For this review, take the finished solid that the model builds, in its own axes (mm). Coordinates: 2 decimals unless noted, no trailing zeros. Write each loop counter-clockwise with the first axis right and the second up, starting at its lowest first coordinate (ties: lowest second). Pieces come first, ordered by that corner, then holes. Notation, with made-up numbers: (72.25, -30) - (106.25, -30) arc R33 ccw to (106.25, -2) - close; hole circle Ø11 at (-37, 2.5). An arc over 180 degrees is marked (long way). Use one line per item in the form item = value. Start each with the question number.
1) Insertion check: P1, Ø1.5, axis at x = -363, z = 7.5, coming from the -Y side; P2, Ø4, axis at y = -68.5, z = 3.5, coming from the +X side. Each pin has a flat end and moves straight along its axis. Give the tip position at first contact, or say it passes through.
2) We need section A-A (z = 9). Give the boundary of the cut face in (x, y), plus the area to 3 significant figures.
3) For L1, parallel to X at y = -31, z = 15; L2, parallel to Y at x = -260, z = 17.5; L3, parallel to X at y = -38, z = 15.5, list the stretches that pass through material, from the lowest coordinate up. Write a range as from..to.
4) We need section B-B (y = -11.5). Give the boundary of the cut face in (x, z).
```python
from build123d import *

# Parameters (mm, degrees)
F0_W     = 685.8
F0_H     = 19.05
F1_DEPTH = 88.9
F3_DEPTH = 127
F5_DEPTH = 127
F7_DEPTH = 25.4


with BuildPart() as f1:
    # F0 (on Front) → F1 (new body)
    with BuildSketch(Plane.XZ):
        with Locations((-342.9, 9.525)):
            Rectangle(F0_W, F0_H)
    extrude(amount=F1_DEPTH)

    # F2 (on face) → F3 (cut)
    with BuildSketch(Plane.XY.offset(19.05)):
        Polygon((0, -88.9), (0, 0), (-62.2484501468, -88.9), align=None)
    extrude(amount=-F3_DEPTH, mode=Mode.SUBTRACT)

    # F4 (on face) → F5 (cut)
    with BuildSketch(Plane.XY.offset(19.05)):
        Polygon((-685.8, 0), (-685.8, -88.9), (-623.5515498532, 0), align=None)
    extrude(amount=-F5_DEPTH, mode=Mode.SUBTRACT)

    # F6 (on face) → F7 (cut)
    with BuildSketch(Plane.XY.offset(19.05)):
        Polygon((-685.8, -88.9), (-62.2484501468, -88.9), (-54.6331555624, -78.0242322185), (-659.9736535614, -52.0161548124), align=None)
    extrude(amount=-F7_DEPTH, mode=Mode.SUBTRACT)


solid = f1.part
```
Determined:
q1.P1 = -64.81
q1.P2 = -46.56
q2.outline = (-659.97, -52.02) - (-54.63, -78.02) - (0, 0) - (-623.55, 0) - close
q2.area = 40,500 mm²
q3.L1 = -645.26..-21.71
q3.L2 = -69.2..0
q3.L3 = -650.16..-26.61
q4.outline = (-631.6, 0) - (-8.05, 0) - (-8.05, 19.05) - (-631.6, 19.05) - close
